Model file for the job. Use its own axes, mm. A direction names the side the tool comes from. Coordinates: 2 decimals unless noted, no trailing zeros. Order: outer loops, then holes, each group sorted by start corner. A loop starts at its lowest first (then second) coordinate and runs counter-clockwise, first axis right, second up.
from build123d import *

# Parameters (mm, degrees)
SKETCH1_W           = 100
SKETCH1_H           = 20
SKETCH1_R           = 3.15
BOSS_EXTRUDE1_DEPTH = 20
SKETCH8_W           = 40
SKETCH8_H           = 20
BOSS_EXTRUDE2_DEPTH = 20
SKETCH9_W           = 19
SKETCH9_H           = 40
CUT_EXTRUDE5_DEPTH  = 20
SKETCH10_R          = 4.1
CUT_EXTRUDE6_DEPTH  = 79.74007874
SKETCH11_W          = 12.4
SKETCH11_H          = 20
BOSS_EXTRUDE3_DEPTH = 30
FILLET1_R           = 10
FILLET2_R           = 5
SKETCH12_R          = 4.1
CUT_EXTRUDE7_DEPTH  = 94.03897033
BOSS_EXTRUDE4_START = 40
SKETCH13_W          = 20
SKETCH13_H          = 20
SKETCH13_R          = 3.15
BOSS_EXTRUDE4_DEPTH = 40
FILLET3_R           = 10
CHAMFER1_SIZE       = 0.5
SKETCH5_R           = 7
CUT_EXTRUDE3_DEPTH  = 50


with BuildPart() as part:
    # Sketch1 → Boss-Extrude1 (new body)
    with BuildSketch(Plane.XY):
        Rectangle(SKETCH1_W, SKETCH1_H)
        with Locations((-40, 0)):
            Circle(SKETCH1_R, mode=Mode.SUBTRACT)
        with Locations((40, 0)):
            Circle(SKETCH1_R, mode=Mode.SUBTRACT)
    extrude(amount=BOSS_EXTRUDE1_DEPTH)

    # Sketch8 → Boss-Extrude2 (add)
    with BuildSketch(Plane(origin=(0, 10, 0), x_dir=(1, 0, 0), z_dir=(0, 1, 0))):
        with Locations((0, -10)):
            Rectangle(SKETCH8_W, SKETCH8_H)
    extrude(amount=BOSS_EXTRUDE2_DEPTH)

    # Sketch9 → Cut-Extrude5 (cut)
    with BuildSketch(Plane(origin=(0, 30, 0), x_dir=(1, 0, 0), z_dir=(0, 1, 0))):
        Rectangle(SKETCH9_W, SKETCH9_H)
    extrude(amount=-CUT_EXTRUDE5_DEPTH, mode=Mode.SUBTRACT)

    # Sketch10 → Cut-Extrude6 (cut, through all)
    with BuildSketch(Plane(origin=(20, 0, 0), x_dir=(0, 0, -1), z_dir=(1, 0, 0))):
        with Locations((-10, 21)):
            Circle(SKETCH10_R)
    extrude(amount=-CUT_EXTRUDE6_DEPTH, mode=Mode.SUBTRACT)

    # Sketch11 → Boss-Extrude3 (add)
    with BuildSketch(Plane.XY.offset(20)):
        with Locations((-16.3, 0)):
            Rectangle(SKETCH11_W, SKETCH11_H)
        with Locations((16.3, 0)):
            Rectangle(SKETCH11_W, SKETCH11_H)
    extrude(amount=BOSS_EXTRUDE3_DEPTH)

    # Fillet1
    # the kernel refuses this fillet: 10 mm, written as the material it adds along each edge
    with BuildSketch(Plane(origin=(-10.1, 10, 20), x_dir=(1, 0, 0), z_dir=(0, -1, 0))) as fillet1_piece_1:
        with BuildLine():
            CenterArc((FILLET1_R, FILLET1_R), FILLET1_R, 180, 90)
            Line((0, FILLET1_R), (0, 0))
            Line((0, 0), (FILLET1_R, 0))
        make_face()
    extrude(amount=20)
    with BuildSketch(Plane(origin=(10.1, 10, 20), x_dir=(-1, 0, 0), z_dir=(0, -1, 0))) as fillet1_piece_2:
        with BuildLine():
            CenterArc((FILLET1_R, -FILLET1_R), FILLET1_R, 90, 90)
            Line((0, -FILLET1_R), (0, 0))
            Line((0, 0), (FILLET1_R, 0))
        make_face()
    extrude(amount=20)

    # Fillet2
    fillet2_edges = [part.edges().sort_by_distance(p)[0] for p in [
        (-22.5, 0, 20),
        (22.5, 0, 20),
    ]]
    fillet(fillet2_edges, radius=FILLET2_R)

    # Sketch12 → Cut-Extrude7 (cut, through all)
    with BuildSketch(Plane(origin=(22.5, 0, 0), x_dir=(0, 0, -1), z_dir=(1, 0, 0))):
        with Locations((-40, 0)):
            Circle(SKETCH12_R)
    extrude(amount=-CUT_EXTRUDE7_DEPTH, mode=Mode.SUBTRACT)

    # Sketch13 → Boss-Extrude4 (add)
    # profile 1 of 2: a face of its own
    with BuildSketch(Plane(origin=(0, 0, 0), x_dir=(-1, 0, 0), z_dir=(0, 0, -1)).offset(BOSS_EXTRUDE4_START)):
        with Locations((-40, 0)):
            Rectangle(SKETCH13_W, SKETCH13_H)
        with Locations((-40, 0)):
            Circle(SKETCH13_R, mode=Mode.SUBTRACT)
    # profile 2 of 2: a face of its own
    with BuildSketch(Plane(origin=(0, 0, 0), x_dir=(-1, 0, 0), z_dir=(0, 0, -1)).offset(BOSS_EXTRUDE4_START)):
        with Locations((40, 0)):
            Rectangle(SKETCH13_W, SKETCH13_H)
        with Locations((40, 0)):
            Circle(SKETCH13_R, mode=Mode.SUBTRACT)
    extrude(amount=-BOSS_EXTRUDE4_DEPTH)

    # Fillet3
    fillet3_edges = [part.edges().sort_by_distance(p)[0] for p in [
        (-30, 0, 0),
        (30, 0, 0),
    ]]
    fillet(fillet3_edges, radius=FILLET3_R)

    # Chamfer1
    chamfer1_edges = [part.edges().sort_by_distance(p)[0] for p in [
        (-7.171067812, -10, 22.928932188),
        (-50, 0, 20),
        (-38.75, 10, 20),
        (38.75, -10, 20),
        (-23.964466094, -10, 21.464466094),
        (-23.964466094, 10, 21.464466094),
        (23.964466094, 10, 21.464466094),
        (23.964466094, -10, 21.464466094),
        (50, 0, -40),
        (40, -10, -40),
        (30, -10, -25),
        (30, 10, -25),
        (-50, 0, -40),
        (-40, -10, -40),
        (-38.75, -10, 20),
        (-30, 10, -25),
        (-30, -10, -25),
        (0, -10, 0),
        (-27.071067812, -10, -2.928932188),
        (-27.071067812, 10, -2.928932188),
        (27.071067812, 10, -2.928932188),
        (27.071067812, -10, -2.928932188),
        (-20, 30, 10),
        (-14.75, 30, 20),
        (20, 30, 10),
        (14.75, 30, 0),
        (14.75, 30, 20),
        (-14.75, 30, 0),
        (-9.5, 30, 10),
        (0, 10, 0),
        (9.5, 20, 0),
        (-9.5, 20, 0),
        (9.5, 10, 10),
        (-9.5, 10, 10),
        (9.5, 30, 10),
        (50, 0, 20),
        (-22.5, 10, 37.5),
        (-22.5, -10, 37.5),
        (-10.1, -10, 40),
        (-10.1, 10, 40),
        (-16.3, -10, 50),
        (50, -10, -10),
        (-50, -10, -10),
        (22.5, -10, 37.5),
        (-50, 10, -10),
        (22.5, 10, 37.5),
        (10.1, 10, 40),
        (50, 10, -10),
        (10.1, -10, 40),
        (16.3, -10, 50),
        (38.75, 10, 20),
        (0, 10, 20),
        (0, -10, 20),
        (7.171067812, -10, 22.928932188),
        (7.171067812, 10, 22.928932188),
        (-7.171067812, 10, 22.928932188),
    ]]
    chamfer(chamfer1_edges, length=CHAMFER1_SIZE)

    # Sketch5 → Cut-Extrude3 (cut)
    with BuildSketch(Plane.XY.offset(20)):
        with Locations((-40, 0)):
            Circle(SKETCH5_R)
        with Locations((40, 0)):
            Circle(SKETCH5_R)
    extrude(amount=-CUT_EXTRUDE3_DEPTH, mode=Mode.SUBTRACT)


solid = part.part
Q1. Probe line 1 (Y direction, x = -13, z = 10); line 2 (X direction, y = 4, z = -11); line 3 (Y direction, x = 40, z = -20). List the from-to ranges inside material, lowest first.
Established:
line 1: y = -10 to 16.9, 25.1 to 30
line 2: x = -50 to -45.74, -34.26 to -30, 30 to 34.26, 45.74 to 50
line 3: y = -10 to -7, 7 to 10
Q2. Mould opens along X. For faces 4 (the face through (-16, 0, 50)), 5 (the face through (10.1, -4.4, 39.9)), 6 (the face through (50, 0, -10)) say: pulls with the +X half, pulls with the -X half, needs draft (parallel to the pull), parting line crosses it, or undercut.
Established:
face 4: needs draft
face 5: undercut
face 6: pulls with the +X half
Q3. Cut at D-D, the plane z = 40. List the corners of the cut face in (x, y).
Established:
outline: (-22.5, -9.5) - (-22, -10) - (-10.6, -10) - (-10.1, -9.5) - (-10.1, -4.1) - (-22.5, -4.1) - close; (-22.5, 4.1) - (-10.1, 4.1) - (-10.1, 9.5) - (-10.6, 10) - (-22, 10) - (-22.5, 9.5) - close; (10.1, -9.5) - (10.6, -10) - (22, -10) - (22.5, -9.5) - (22.5, -4.1) - (10.1, -4.1) - close; (10.1, 4.1) - (22.5, 4.1) - (22.5, 9.5) - (22, 10) - (10.6, 10) - (10.1, 9.5) - close
Q4. Cut at B-B, the plane z = -14. List the corners of the cut face in (x, y).
Established:
outline: (-50, -9.5) - (-49.5, -10) - (-30.5, -10) - (-30, -9.5) - (-30, 9.5) - (-30.5, 10) - (-49.5, 10) - (-50, 9.5) - close; (30, -9.5) - (30.5, -10) - (49.5, -10) - (50, -9.5) - (50, 9.5) - (49.5, 10) - (30.5, 10) - (30, 9.5) - close; hole circle Ø14 at (-40, 0); hole circle Ø14 at (40, 0)
Q5. Which spindle directions (+Z, -Z, +X, -X, +Y, -Y) get a long thin tool onto all of the face, cutting with end or side? Do faces 1 (the face through (27.25, 9.64, -2.91)), 2 (the face through (-26.99, 0.13, -2.85)), 3 (the face through (7.19, -9.64, 22.75)). Say none if no direction does.
Established:
face 1: -Z, +Y
face 2: -Z, +Y, -Y
face 3: +Z, -Y
Q6. Cut at A-A, the plane z = 10. Count the separate pieces of the cut face and the enclosed holes in it, plus the area to 3 significant figures.
Established:
separate pieces: 3
enclosed holes: 2
area: 1,940 mm2
Q7. Drop flat-ended pins along their axis: P1, Ø12, axis at x = 13.5, y = 18.5, coming from the +Z side; P2, Ø2, axis at y = 10.5, z = 20, coming from the +X side; P3, Ø8, axis at x = 40, y = 0, coming from the +Z side; P4, Ø6.5, axis at y = 21, z = 10, coming from the +X side. Give the stop position or say it passes through.
Established:
P1: stops at z = 20
P2: stops at x = 49.87
P3: stops at z = -30
P4: passes through
Q8. Cut at C-C, the plane x = -40. List the corners of the cut face in (y, z), plus the area to 3 significant figures.
Established:
outline: (-10, -39.5) - (-9.5, -40) - (-3.15, -40) - (-3.15, -30) - (-7, -30) - (-7, 20) - (-9.5, 20) - (-10, 19.5) - close; (3.15, -40) - (10, -40) - (10, 19.5) - (9.5, 20) - (7, 20) - (7, -30) - (3.15, -30) - close
area: 437 mm2
